Source: CAD feature listing. Evaluate the final solid. Frame: model axes, mm. Face numbers are marked on the shaded views. A direction names the side the tool comes from. Round coordinates to 2 decimals unless told otherwise and drop trailing zeros. Order: outer loops, then holes, each group sorted by start corner. A loop starts at its lowest first (then second) coordinate and runs counter-clockwise, first axis right, second up. Notation, with made-up numbers: (-15, 56) -> (-4, 56) arc R6 cw to (-4, 62) -> close; hole circle Ø11 at (5.5, 32). An arc over 180 degrees is marked (long way). Write item = value, one per line. Start each with the question number.
(1) Reachability of the marked faces 4 and 5 from +Z, -Z, +X, -X, +Y, -Y: full face, straight path, thin tool, end or side. Return the list, or none.
(2) Draft query along Y for the marked faces 1, 2 and 3. Return one class per face: released by +Y, released by -Y, zero draft, split by the parting line, or undercut.
(3) Cut plane B-B on z = 1.25. Return the cut outline in (x, y) (3 decimals).
(4) Contact query for a flat-ended pin moving along its axis: pin 1 Ø3 at (x, y) = (-15.5, 5.5) entering from -Z. Output: stop coordinate, or through.
(5) Ray query, line 1 (Y direction, x = -7.25, z = 3) (3 decimals); line 2 (X direction, y = 7, z = 2.75); line 3 (Z direction, x = -17.5, y = 7). Return the intervals inside material, ascending.
(6) Cut plane C-C on x = -11.25. Return the cut outline in (y, z) (3 decimals).
(7) Cut plane A-A on y = 6.5. Return the cut outline in (x, z), then the cut area to 3 significant figures.
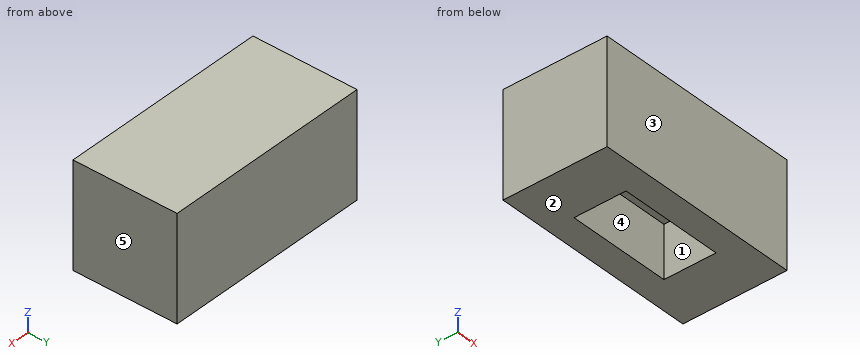
from build123d import *

# Parameters (mm, degrees)
SKETCH1_W           = 25.4
SKETCH1_H           = 12.7
SKETCH1_W_2         = 12.7
SKETCH1_H_2         = 6.35
BOSS_EXTRUDE1_DEPTH = 12.7
SKETCH2_W           = 12.7
SKETCH2_H           = 6.35
BOSS_EXTRUDE2_DEPTH = 6.35


with BuildPart() as part:
    # Sketch1 → Boss-Extrude1 (new body)
    with BuildSketch(Plane.XY):
        with Locations((-12.7, 6.35)):
            Rectangle(SKETCH1_W, SKETCH1_H)
        with Locations((-12.7, 6.35)):
            Rectangle(SKETCH1_W_2, SKETCH1_H_2, mode=Mode.SUBTRACT)
    extrude(amount=BOSS_EXTRUDE1_DEPTH)

    # Sketch2 → Boss-Extrude2 (add)
    with BuildSketch(Plane.XY.offset(12.7)):
        with Locations((-12.7, 6.35)):
            Rectangle(SKETCH2_W, SKETCH2_H)
    extrude(amount=-BOSS_EXTRUDE2_DEPTH)


solid = part.part
Evaluation:
q1.face_4 = -Z
q1.face_5 = +Z, -Z, +X, +Y, -Y
q2.face_1 = undercut
q2.face_2 = zero draft
q2.face_3 = released by -Y
q3.outline = (-25.4, 0) -> (0, 0) -> (0, 12.7) -> (-25.4, 12.7) -> close; hole (-19.05, 3.175) -> (-6.35, 3.175) -> (-6.35, 9.525) -> (-19.05, 9.525) -> close
q4.pin_1 = 6.35
q5.line_1 = 0 to 3.175, 9.525 to 12.7
q5.line_2 = -25.4 to -19.05, -6.35 to 0
q5.line_3 = 6.35 to 12.7
q6.outline = (0, 0) -> (3.175, 0) -> (3.175, 6.35) -> (9.525, 6.35) -> (9.525, 0) -> (12.7, 0) -> (12.7, 12.7) -> (0, 12.7) -> close
q7.outline = (-25.4, 0) -> (-19.05, 0) -> (-19.05, 6.35) -> (-6.35, 6.35) -> (-6.35, 0) -> (0, 0) -> (0, 12.7) -> (-25.4, 12.7) -> close
q7.area = 242 mm^2
